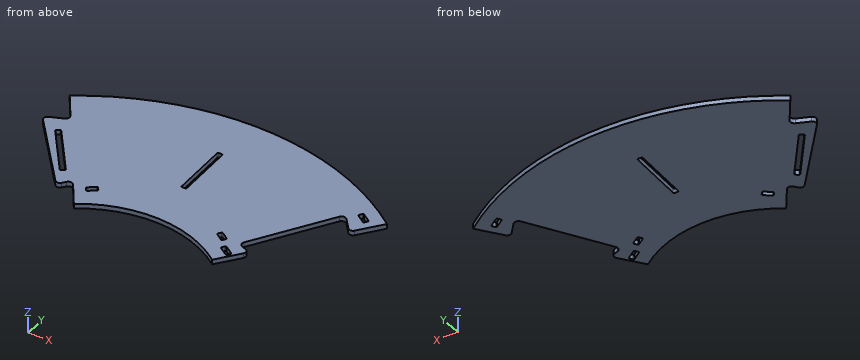
Autodesk Inventor part; units mm, degrees
ref_plane "YZ Plane" through (0, 0, 0) normal (1, 0, 0) x (0, 1, 0)
ref_plane "XZ Plane" through (0, 0, 0) normal (0, 1, 0) x (-1, 0, 0)
ref_plane "XY Plane" through (0, 0, 0) normal (0, 0, 1) x (1, 0, 0)
sketch "Sketch1" plane through (0, 0, 0) normal (0, 0, 1) x (1, 0, 0)
  point P0 (0, 0)
sketch "CONTOURS" plane through (0, 0, 0) normal (0, 0, 1) x (1, 0, 0)
  arc A0 (1138.7708, 133.0427) -> (1131.5929, 155.3323) centre (1127.04, 141.5656) ccw
  line L0 (1131.5929, 155.3323) -> (1115.5781, 160.6286)
  arc A1 (1107.0938, 183.2185) -> (1115.5781, 160.6286) centre (1120.445, 175.3447) ccw
  line L1 (1107.0938, 183.2185) -> (1274.33, 466.7921)
  arc A2 (1299.254, 469.2294) -> (1274.33, 466.7921) centre (1287.6812, 458.9183) ccw
  line L2 (1299.254, 469.2294) -> (1333.4216, 430.8808)
  arc A3 (1333.4216, 430.8808) -> (1355.9785, 432.0038) centre (1344.2478, 440.5267) ccw
  line L3 (1355.9785, 432.0038) -> (1419.4157, 519.3176)
  arc A4 (1419.4157, 519.3176) -> (208.109, 519.3881) centre (813.7138, -315.0977) ccw
  line L4 (208.109, 519.3881) -> (271.5978, 432.0034)
  arc A5 (265.2883, 408.6999) -> (271.5978, 432.0034) centre (259.0581, 422.8927) ccw
  line L5 (265.2883, 408.6999) -> (218.2583, 388.055)
  arc A6 (218.2583, 388.055) -> (213.2217, 365.1756) centre (224.0866, 374.778) ccw
  line L6 (213.2217, 365.1756) -> (431.2374, 118.4955)
  arc A7 (431.2374, 118.4955) -> (453.7882, 119.5137) centre (442.1023, 128.0978) ccw
  line L7 (453.7882, 119.5137) -> (463.7742, 133.108)
  arc A8 (488.8058, 133.0425) -> (463.7742, 133.108) centre (476.2661, 123.9318) ccw
  line L8 (488.8058, 133.0425) -> (549.6876, 49.246)
  arc A9 (1077.8891, 49.2462) -> (549.6876, 49.246) centre (813.7885, -315.108) ccw
  line L9 (1077.8891, 49.2462) -> (1138.7708, 133.0427)
sketch "HOLES" plane through (0, 0, 0) normal (0, 0, 1) x (1, 0, 0)
  line L0 (287.205, 350.9682) -> (278.6203, 344.0905)
  arc A0 (278.6203, 344.0905) -> (277.9995, 338.4678) centre (281.1212, 340.9688) ccw
  line L1 (277.9995, 338.4678) -> (408.6757, 175.3582)
  arc A1 (408.6757, 175.3582) -> (414.2984, 174.7375) centre (411.7974, 177.8592) ccw
  line L2 (414.2984, 174.7375) -> (422.8831, 181.6152)
  arc A2 (422.8831, 181.6152) -> (423.5039, 187.2379) centre (420.3822, 184.7369) ccw
  line L3 (423.5039, 187.2379) -> (292.8277, 350.3475)
  arc A3 (292.8277, 350.3475) -> (287.205, 350.9682) centre (289.706, 347.8465) ccw
  arc A4 (783.5127, 529.4978) -> (779.3287, 533.3049) centre (779.5172, 529.3094) ccw
  line L4 (783.5127, 529.4978) -> (793.3586, 320.7299)
  arc A5 (789.5515, 316.5459) -> (793.3586, 320.7299) centre (789.363, 320.5414) ccw
  line L5 (789.5515, 316.5459) -> (778.5637, 316.0277)
  arc A6 (774.3797, 319.8348) -> (778.5637, 316.0277) centre (778.3752, 320.0232) ccw
  line L6 (774.3797, 319.8348) -> (764.5338, 528.6027)
  arc A7 (768.3409, 532.7867) -> (764.5338, 528.6027) centre (768.5294, 528.7912) ccw
  line L7 (768.3409, 532.7867) -> (779.3287, 533.3049)
  line L8 (569.7888, 155.0903) -> (562.9111, 163.675)
  arc A8 (562.9111, 163.675) -> (557.2884, 164.2957) centre (559.7894, 161.174) ccw
  line L9 (557.2884, 164.2957) -> (533.8755, 145.5384)
  arc A9 (533.8755, 145.5384) -> (533.2548, 139.9157) centre (536.3765, 142.4167) ccw
  line L10 (533.2548, 139.9157) -> (540.1325, 131.331)
  arc A10 (540.1325, 131.331) -> (545.7552, 130.7102) centre (543.2542, 133.832) ccw
  line L11 (545.7552, 130.7102) -> (569.168, 149.4676)
  arc A11 (569.168, 149.4676) -> (569.7888, 155.0903) centre (566.6671, 152.5893) ccw
  line L12 (1012.5411, 175.9713) -> (1018.5803, 185.1652)
  arc A12 (1024.1197, 186.3123) -> (1018.5803, 185.1652) centre (1021.9236, 182.9691) ccw
  line L13 (1024.1197, 186.3123) -> (1049.1939, 169.8417)
  arc A13 (1050.3411, 164.3024) -> (1049.1939, 169.8417) centre (1046.9978, 166.4985) ccw
  line L14 (1059.1699, 932.849) -> (1052.9484, 923.7775)
  arc A14 (1047.3873, 922.7411) -> (1052.9484, 923.7775) centre (1049.6497, 926.0399) ccw
  line L15 (1047.3873, 922.7411) -> (1017.6987, 943.1026)
  arc A15 (1016.6623, 948.6637) -> (1017.6987, 943.1026) centre (1019.9611, 946.4013) ccw
  line L16 (1016.6623, 948.6637) -> (1022.8839, 957.7352)
  arc A16 (1028.445, 958.7715) -> (1022.8839, 957.7352) centre (1026.1826, 955.4728) ccw
  line L17 (1028.445, 958.7715) -> (1058.1336, 938.4101)
  arc A17 (1059.1699, 932.849) -> (1058.1336, 938.4101) centre (1055.8712, 935.1114) ccw
  arc A18 (2370.6146, 1037.7855) -> (2376.2246, 1037.059) centre (2373.7829, 1040.2273) ccw
  line L18 (2370.6146, 1037.7855) -> (2296.1408, 1134.417)
  arc A19 (2296.8672, 1140.027) -> (2296.1408, 1134.417) centre (2299.309, 1136.8588) ccw
  line L19 (2296.8672, 1140.027) -> (2305.5799, 1146.7419)
  arc A20 (2311.1899, 1146.0154) -> (2305.5799, 1146.7419) centre (2308.0217, 1143.5736) ccw
  line L20 (2311.1899, 1146.0154) -> (2385.6638, 1049.3839)
  arc A21 (2384.9373, 1043.7739) -> (2385.6638, 1049.3839) centre (2382.4955, 1046.9421) ccw
  line L21 (2384.9373, 1043.7739) -> (2376.2246, 1037.059)
  line L22 (1175.8209, 1180.7295) -> (1169.5993, 1171.658)
  arc A22 (1169.5993, 1171.658) -> (1170.6357, 1166.0969) centre (1172.898, 1169.3956) ccw
  line L23 (1170.6357, 1166.0969) -> (1200.3242, 1145.7355)
  arc A23 (1200.3242, 1145.7355) -> (1205.8854, 1146.7718) centre (1202.5866, 1149.0342) ccw
  line L24 (1205.8854, 1146.7718) -> (1212.1069, 1155.8433)
  arc A24 (1212.1069, 1155.8433) -> (1211.0706, 1161.4044) centre (1208.8082, 1158.1057) ccw
  line L25 (1211.0706, 1161.4044) -> (1181.382, 1181.7659)
  arc A25 (1181.382, 1181.7659) -> (1175.8209, 1180.7295) centre (1179.1196, 1178.4671) ccw
  line L26 (1050.3411, 164.3024) -> (1044.3019, 155.1085)
  arc A26 (1038.7625, 153.9613) -> (1044.3019, 155.1085) centre (1040.9586, 157.3046) ccw
  line L27 (1038.7625, 153.9613) -> (1013.6883, 170.4319)
  arc A27 (1012.5411, 175.9713) -> (1013.6883, 170.4319) centre (1015.8843, 173.7752) ccw
  line L28 (1101.0619, 97.7126) -> (1107.1011, 106.9065)
  arc A28 (1107.1011, 106.9065) -> (1105.954, 112.4458) centre (1103.7579, 109.1026) ccw
  line L29 (1105.954, 112.4458) -> (1075.8649, 132.2106)
  arc A29 (1075.8649, 132.2106) -> (1070.3255, 131.0634) centre (1073.6688, 128.8673) ccw
  line L30 (1070.3255, 131.0634) -> (1064.2863, 121.8695)
  arc A30 (1064.2863, 121.8695) -> (1065.4335, 116.3302) centre (1067.6295, 119.6734) ccw
  line L31 (1065.4335, 116.3302) -> (1095.5226, 96.5655)
  arc A31 (1095.5226, 96.5655) -> (1101.0619, 97.7126) centre (1097.7187, 99.9087) ccw
  line L32 (1362.3431, 495.4778) -> (1356.3039, 486.2839)
  arc A32 (1350.7646, 485.1368) -> (1356.3039, 486.2839) centre (1352.9607, 488.48) ccw
  line L33 (1350.7646, 485.1368) -> (1320.6755, 504.9015)
  arc A33 (1319.5283, 510.4408) -> (1320.6755, 504.9015) centre (1322.8716, 508.2448) ccw
  line L34 (1319.5283, 510.4408) -> (1325.5675, 519.6347)
  arc A34 (1331.1069, 520.7819) -> (1325.5675, 519.6347) centre (1328.9108, 517.4387) ccw
  line L35 (1331.1069, 520.7819) -> (1361.196, 501.0172)
  arc A35 (1362.3431, 495.4778) -> (1361.196, 501.0172) centre (1358.9999, 497.6739) ccw
  line L36 (1264.9795, 244.1751) -> (1271.0187, 253.369)
  arc A36 (1276.558, 254.5161) -> (1271.0187, 253.369) centre (1274.3619, 251.1729) ccw
  line L37 (1276.558, 254.5161) -> (1306.6471, 234.7514)
  arc A37 (1307.7943, 229.2121) -> (1306.6471, 234.7514) centre (1304.451, 231.4082) ccw
  line L38 (1307.7943, 229.2121) -> (1301.7551, 220.0182)
  arc A38 (1296.2157, 218.871) -> (1301.7551, 220.0182) centre (1298.4118, 222.2143) ccw
  line L39 (1296.2157, 218.871) -> (1266.1266, 238.6358)
  arc A39 (1264.9795, 244.1751) -> (1266.1266, 238.6358) centre (1268.3227, 241.979) ccw
  line L40 (1526.2607, 641.9403) -> (1520.2215, 632.7464)
  arc A40 (1520.2215, 632.7464) -> (1521.3686, 627.2071) centre (1523.5647, 630.5503) ccw
  line L41 (1521.3686, 627.2071) -> (1551.4577, 607.4424)
  arc A41 (1551.4577, 607.4424) -> (1556.9971, 608.5895) centre (1553.6538, 610.7856) ccw
  line L42 (1556.9971, 608.5895) -> (1563.0363, 617.7834)
  arc A42 (1563.0363, 617.7834) -> (1561.8891, 623.3227) centre (1559.6931, 619.9795) ccw
  line L43 (1561.8891, 623.3227) -> (1531.8, 643.0875)
  arc A43 (1531.8, 643.0875) -> (1526.2607, 641.9403) centre (1529.6039, 639.7442) ccw
sketch "LETTERS" plane through (0, 0, 0) normal (0, 0, 1) x (1, 0, 0)
  arc A0 (1107.5534, 367.1718) -> (1103.7785, 359.006) centre (1105.6754, 363.0845) ccw
  line L0 (1107.5534, 367.1718) -> (1115.5892, 363.4795)
  arc A1 (1112.0249, 376.8584) -> (1107.5534, 367.1718) centre (1109.7806, 372.0191) ccw
  line L1 (1120.1257, 373.1016) -> (1112.0249, 376.8584)
  line L2 (1111.8629, 355.2459) -> (1120.1257, 373.1016)
  line L3 (1103.7785, 359.006) -> (1111.8629, 355.2459)
extrude "Extrusion2" add sketch "CONTOURS" along normal blind 18
extrude "Extrusion3" cut sketch "HOLES" along normal through all contours A3 L3 A2 L2 A1 L1 A0 L0 | L4 A5 L5 A6 L6 A7 L7 A4 | A11 L11 A10 L10 A9 L9 A8 L8 | L12 A12 L13 A13 L26 A26 L27 A27 | A31 L31 A30 L30 A29 L29 A28 L28 | L32 A32 L33 A33 L34 A34 L35 A35
properties part number "Platform B3" material "Wood (Birch)"
Geometry check sheet. Reference: the model listing, model coordinates, mm. Give positions to 0.01 mm unless a question says otherwise; leave off trailing zeros. Order: outer loops, then holes, each group sorted by start corner. A loop starts at its lowest first (then second) coordinate and runs counter-clockwise, first axis right, second up. Notation, with made-up numbers: M 39,14.25 L 75,14.25 A10 cw 75,18.25 Z; hole C 2.5,78.5 d10. An arc over 180 degrees is marked long. Use a Markdown table: item, result.
Item 1: Material ranges on line 1 along X through (y, z) = (350.5, 6.75); line 2 along X through (y, z) = (258, 16.75); line 3 along X through (y, z) = (192, 13), recorded low to high.
Answers follow:
| item | result |
|---|---|
| line 1 | x = 226.19 to 286.62, 292.7 to 772.93, 791.95 to 1205.75 |
| line 2 | x = 307.94 to 342.47, 366.81 to 1151.2 |
| line 3 | x = 366.27 to 395.34, 419.69 to 1112.27 |
Item 2: Section check C-C (y = 664). Record the cut outline in (x, z).
Answers follow:
| item | result |
|---|---|
| outline | M 490.46,0 L 1136.97,0 L 1136.97,18 L 490.46,18 Z |
Item 3: Depth check by flat-ended pin: P1, Ø8, axis at y = 190, z = 14.5, coming from the +X side; P2, Ø8, axis at y = 495, z = 11.5, coming from the +X side; P3, Ø4, axis at y = 347.5, z = 10, coming from the +X side; P4, Ø5, axis at x = 497, y = 403, coming from the -Z side. Enter the tip coordinate at first touch or a pass-through.
Answers follow:
| item | result |
|---|---|
| P1 | stops at x = 1113.45 |
| P2 | stops at x = 1404.65 |
| P3 | stops at x = 1205.16 |
| P4 | stops at z = 0 |
Item 4: Section check B-B (x = 1239.5). Record the cut outline in (y, z).
Answers follow:
| item | result |
|---|---|
| outline | M 407.73,0 L 623.96,0 L 623.96,18 L 407.73,18 Z |
Item 5: Section check A-A (z = 3.5). State how many separate pieces and enclosed holes the cut face has, and give its area (3 significant figures).
Answers follow:
| item | result |
|---|---|
| separate pieces | 1 |
| enclosed holes | 6 |
| area | 529,000 mm2 |
